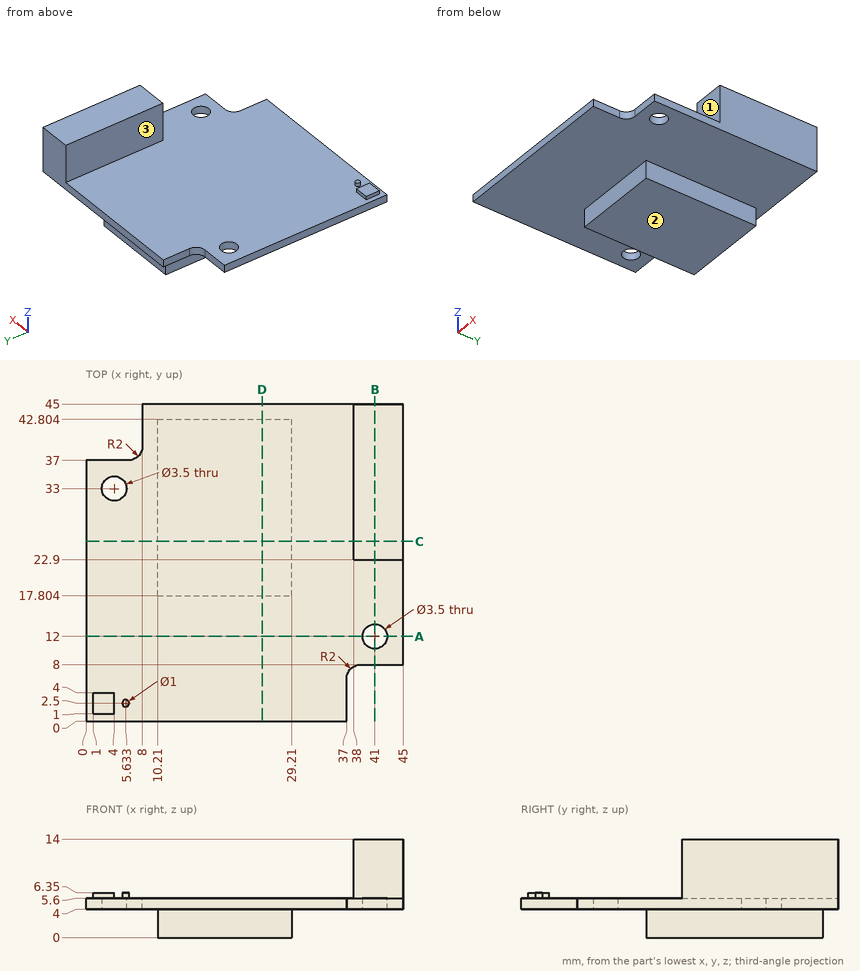
Source: three-view drawing plus pictorial views. Frame: mm from the lowest corner of the part. A direction names the side the tool comes from. Give positions to 0.01 mm unless a question says otherwise; leave off trailing zeros. Loops run counter-clockwise (first coordinate to the right, second up) from the corner with the lowest first, then second, coordinate; pieces in that order, holes last.
1) Section query A-A on y = 12. Return the cut outline in (x, z).
A:
outline: (0, 4) - (39.25, 4) - (39.25, 5.6) - (0, 5.6) - close; (42.75, 4) - (45, 4) - (45, 5.6) - (42.75, 5.6) - close
2) Line query: L1, parallel to X at y = 12, z = 4.5; L2, parallel to Y at x = 4, z = 4.7; L3, parallel to Y at x = 41, z = 5.2. Output: solid intervals per line, ascending.
A:
L1: x = 0 to 39.25, 42.75 to 45
L2: y = 0 to 31.25, 34.75 to 37
L3: y = 8 to 10.25, 13.75 to 45
3) Contact query for flat-ended pins moving along their axis: pin 1 (4.5 mm diameter, centred on x = 41, y = 12, fed in from +Z); pin 2 (0.6 mm diameter, centred on y = 2, z = 6, fed in from +X); pin 3 (2 mm diameter, centred on x = 16, z = 2, fed in from +Y). Output: stop coordinate, or through.
A:
pin 1: stops at z = 5.6
pin 2: stops at x = 6.09
pin 3: stops at y = 42.8
4) Section query D-D on x = 25. Return the cut outline in (y, z), and give its area (3 significant figures).
A:
outline: (0, 4) - (17.8, 4) - (17.8, 0) - (42.8, 0) - (42.8, 4) - (45, 4) - (45, 5.6) - (0, 5.6) - close
area: 172 mm2
5) Section query B-B on x = 41. Return the cut outline in (y, z), and give its area (3 significant figures).
A:
outline: (8, 4) - (10.25, 4) - (10.25, 5.6) - (8, 5.6) - close; (13.75, 4) - (45, 4) - (45, 14) - (22.9, 14) - (22.9, 5.6) - (13.75, 5.6) - close
area: 239 mm2
6) Reachability of the marked faces 1, 2 and 3 from +Z, -Z, +X, -X, +Y, -Y: full face, straight path, thin tool, end or side. Return the list, or none.
A:
face 1: +Z, +X, -X, -Y
face 2: -Z, +X, -X, +Y, -Y
face 3: +Z, -X, +Y, -Y
7) Section query C-C on y = 25.5. Return the cut outline in (x, z), and give its area (3 significant figures).
A:
outline: (0, 4) - (10.21, 4) - (10.21, 0) - (29.21, 0) - (29.21, 4) - (45, 4) - (45, 14) - (38, 14) - (38, 5.6) - (0, 5.6) - close
area: 207 mm2
